The model under review builds one solid part; all positions refer to its coordinate system, in mm. A direction names the side the tool comes from. Give positions to 0.01 mm unless a question says otherwise; leave off trailing zeros. Order: outer loops, then holes, each group sorted by start corner. A loop starts at its lowest first (then second) coordinate and runs counter-clockwise, first axis right, second up. Notation, with made-up numbers: (-31, 6) - (-7, 6) arc R22 ccw to (-7, 12) - close; hole circle Ø6 at (88, 68.5). An arc over 180 degrees is marked (long way). Put each result on its own line as item: value.
Autodesk Inventor part; units mm, degrees
ref_plane "Work Plane1" through (-52.254036, 0, 0.064657) normal (1, 0, 0) x (0, 0, -1)
ref_plane "YZ Plane" through (0, 0, 0) normal (1, 0, 0) x (0, 1, 0)
ref_plane "XZ Plane" through (0, 0, 0) normal (0, 1, 0) x (-1, 0, 0)
sketch "Sketch1" plane through (0, 0, 0) normal (0, 1, 0) x (-1, 0, 0)
  circle A0 centre (18.719305, 0.91995) radius 3.625
  line L0 (19.118903, 4.522858) -> (19.118903, 6.41995)
  line L1 (19.118903, 6.41995) -> (18.491054, 7.168191)
  line L2 (18.491054, 7.168191) -> (20.291054, 8.668191)
  line L3 (20.291054, 8.668191) -> (21.541054, 8.418191)
  line L4 (21.541054, 8.418191) -> (22.541054, 7.418191)
  line L5 (22.541054, 7.418191) -> (26.041054, 5.418191)
  line L6 (26.041054, -4.16305) -> (26.041054, 5.418191)
  line L7 (26.041054, 5.418191) -> (45.041054, 5.418191)
  line L8 (45.041054, 5.418191) -> (49.279808, 4.102266)
  line L9 (18.849216, -2.702721) -> (26.041054, -2.702721)
  circle A1 centre (48.026329, 0.064657) radius 4.227707
  line L10 (48.026329, -4.16305) -> (26.041054, -4.16305)
  circle A2 centre (18.719305, 0.91995) radius 3
  point P0 (0, 0)
  dimension "d0" = 7.25
  dimension "d1" = 5.5
  dimension "d2" = 140
  dimension "d3" = 1.5
  dimension "d4" = 1.8
  dimension "d5" = 1.25
  dimension "d6" = 0.25
  dimension "d7" = 1
  dimension "d8" = 1
  dimension "d9" = 3.5
  dimension "d10" = 2
  dimension "d11" = 19
  dimension "d12" = 6
  dimension "d15" = 5.083
extrude "Extrusion1" add sketch "Sketch1" along normal mid plane 5.95
ref_plane "Work Plane1" through (-52.254036, 0, 0.064657) normal (1, 0, 0) x (0, 0, -1)
sketch "Sketch2" plane through (-52.254036, 0, 0.064657) normal (1, 0, 0) x (0, 0, -1)
  point P0 (0.064657, 0)
sketch "Sketch3" plane through (-52.254036, 0, 0.064657) normal (1, 0, 0) x (0, 0, -1)
  line L0 (-4.03761, -2.975) -> (4.227707, -2.975) construction
  line L1 (4.227707, 2.975) -> (-4.03761, 2.975) construction
  line L2 (-4.03761, -2.975) -> (-4.03761, 2.975) construction
  line L3 (2.767378, 2.975) -> (4.227707, 2.975) construction
  line L4 (-4.03761, -2.975) -> (4.227707, 2.975) construction
  line L5 (4.227707, -2.975) -> (4.227707, 2.975) construction
  line L6 (4.227707, -2.975) -> (0.095048, 0) construction
  line L7 (-3.654952, -2.5) -> (3.845048, -2.5)
  line L8 (3.845048, -2.5) -> (3.845048, 2.5)
  line L9 (3.845048, 2.5) -> (-3.654952, 2.5)
  line L10 (-3.654952, 2.5) -> (-3.654952, -2.5)
  line L11 (-3.654952, -2.5) -> (3.845048, 2.5) construction
  line L12 (3.845048, -2.5) -> (-3.654952, 2.5) construction
  point P0 (0.064657, 0)
  dimension "d16" = 7.5
  dimension "d17" = 5
extrude "Extrusion2" cut sketch "Sketch3" along normal blind 8.25
sketch "Sketch4" plane through (-50.151142, -2.5, 3.719608) normal (0, 1, 0) x (1, 0, 0)
  arc A0 (2.124813, 7.882658) -> (0.871334, -0.382658) centre (2.124813, 3.654952) ccw
  circle A1 centre (2.124813, 3.654952) radius 2.55
  point P0 (50.151142, 3.719608)
  dimension "d20" = 5.1
extrude "Extrusion3" add sketch "Sketch4" along normal up to surface (5 mm away)
sketch "Sketch5" plane through (-49.783914, -2.5, -3.780392) normal (0, 0, 1) x (1, 0, 0)
  line L0 (0, 0) -> (0, 5)
  line L1 (0, 0) -> (3.5, 0)
  line L2 (3.5, 0) -> (3.5, 5)
  line L3 (0, 5) -> (3.5, 5)
  point P0 (49.783914, 2.5)
  point P1 (3.5, 0.293722)
  dimension "d23" = 3.5
extrude "Extrusion4" cut sketch "Sketch5" against normal blind 4.25
sketch "Sketch6" plane through (-44.004036, 2.5, 3.719608) normal (0, 0, -1) x (-1, 0, 0)
  line L0 (6.147107, 0) -> (0, 0)
  line L1 (6.147107, 0) -> (4.147107, 0)
  line L2 (4.147107, 0) -> (4.147107, -5)
  line L3 (4.147107, -5) -> (6.147107, -5)
  line L4 (6.147107, -5) -> (6.147107, 0)
  line L5 (6.147107, -5) -> (0, -5)
  point P0 (-44.004036, -2.5)
  point P1 (4.147107, 0)
  dimension "d26" = 2
extrude "Extrusion5" cut sketch "Sketch6" against normal blind 4.25
fillet "Fillet1" radius 0.3665 2 edges at (-48.1511, 0, 4.4527) (-48.1511, 0, 3.7196)
chamfer "Chamfer1" distance 0.5 angle 45 8 edges at (-35.5411, -2.975, 5.4182) (-35.5411, 2.975, 5.4182) (-24.2911, 2.975, 6.4182) (-24.2911, -2.975, 6.4182) (-22.0411, -2.975, 7.9182) (-22.0411, 2.975, 7.9182) (-20.9161, 2.975, 8.5432) (-20.9161, -2.975, 8.5432)
chamfer "Chamfer2" distance 1 angle 45 1 edges at (-26.0411, 0, -4.1631)
properties part number "Lower Leg"
(1) Take a section at A-A, the plane y = 1.45. Count the separate pieces of the cut face and the enclosed holes in it, then the cut area to 3 significant figures.
The answers:
separate pieces: 2
enclosed holes: 1
area: 263 mm^2
(2) Clearance check with flat-ended pins moving along their axes: pin 1 Ø1.5 at (y, z) = (-2, 0) entering from +X; pin 2 Ø2.5 at (x, y) = (-45.5, 1) entering from +Z; pin 3 Ø0.9 at (y, z) = (1, 5.5) entering from +X; pin 4 Ø5 at (x, z) = (-18.72, 0.92) entering from +Y. State where each tip first meets the part, or that it passes through.
The answers:
pin 1: x = -15.1
pin 2: z = 5.42
pin 3: x = -19.12
pin 4: through
(3) Take a section at D-D, the plane x = -37. Write out the cut boundary in (y, z) (3 decimals), then the cut area to 3 significant figures.
The answers:
outline: (-2.975, -4.163) - (2.975, -4.163) - (2.975, 4.918) - (2.475, 5.418) - (-2.475, 5.418) - (-2.975, 4.918) - close
area: 56.8 mm^2
(4) For faces 1 (the flat face through (-35, 0, 5.418)), 2 (the flat face through (-22, 0, -2.703)), 3 (the flat face through (-45, 0, -3.78)), list the 3-axis set-ups (+Z, -Z, +X, -X, +Y, -Y) from which the entire face can be reached by the end or side of a thin tool; tool diameter is ignored.
The answers:
face 1: +Z, -X, +Y, -Y
face 2: -Z, +X, +Y, -Y
face 3: -X
(5) Take a section at C-C, the plane z = 3. Write out the cut boundary in (x, y) (1 decimal).
The answers:
outline: (-51.1, -3) - (-20.9, -3) - (-20.9, 3) - (-51.1, 3) - (-51.1, 2.5) - (-44, 2.5) - (-44, -2.5) - (-51.1, -2.5) - close; (-16.6, -3) - (-15.8, -3) - (-15.8, 3) - (-16.6, 3) - close
(6) The part is to be moulded in two halves that separate along X. For faces 4 (the cylindrical face through (-45.594, -0.035, 0.831)), 5 (the flat face through (-24.172, 2.721, 6.203)), 6 (the flat face through (-46, 0, 3.72)), 7 (the flat face through (-45, -2.5, 0)), say which applies: pulls with the +X half, pulls with the -X half, needs draft (parallel to the pull), parting line crosses it, or undercut.
The answers:
face 4: undercut
face 5: pulls with the -X half
face 6: needs draft
face 7: undercut
(7) Wall thickness on L1, parallel to Y at x = -46, z = 3 (3 decimals); L2, parallel to X at y = -2.2, z = -1.25; L3, parallel to Z at x = -38.5, y = -2.25: over which ranges is each line inside the solid? List them lowest first.
The answers:
L1: -2.975 to -2.5, 2.5 to 2.975
L2: -50.21 to -45.84, -44 to -20.79, -16.65 to -15.82
L3: -4.16 to 5.42
(8) Take a section at B-B, the plane z = -0.75. Write out the cut boundary in (x, y) (3 decimals).
The answers:
outline: (-52.175, -2.975) - (-21.212, -2.975) - (-21.212, 2.975) - (-52.175, 2.975) - (-52.175, 2.5) - (-50.443, 2.5) - (-50.443, -2.5) - (-52.175, -2.5) - close; (-16.227, -2.975) - (-15.502, -2.975) - (-15.502, 2.975) - (-16.227, 2.975) - close; hole (-45.61, -2.5) - (-44.004, -2.5) - (-44.004, 2.5) - (-45.61, 2.5) - close
